from build123d import *

# Parameters (mm, degrees)
ESQUISSE1_W                               = 256
ESQUISSE1_H                               = 100
T_LE_DE_BASE_PLI_E1_DEPTH                 = 10
ESQUISSE15_W                              = 256
ESQUISSE15_H                              = 10
BOSS_EXTRU_3_DEPTH                        = 10
ENL_V_MAT_EXTRU_1_REACH                   = 277.02
ESQUISSE9_R                               = 39
SKETCH7_W                                 = 10
SKETCH7_H                                 = 55
EXTRUDE2_DEPTH                            = 10
SKETCH8_W                                 = 40
SKETCH8_H                                 = 200
EXTRUDE3_DEPTH                            = 10
ESQUISSE11_W                              = 15
ESQUISSE11_H                              = 10
BOSS_EXTRU_2_DEPTH                        = 10
TROU_POUR_TARAUDAGE_POUR_TROU_TARAUD_M1_D = 14
CHANFREIN1_SIZE                           = 2
TAB_START                                 = -10
TAB_AND_SLOT_TAB1_DEPTH                   = 10
DIAM_TRE_DU_PER_AGE_2_0_2_1_D             = 2
ENL_V_START                               = -10
ESQUISSE19_W                              = 78
ESQUISSE19_H                              = 10
ENL_V_MAT_EXTRU_2_DEPTH                   = 10


# Read off the part's stored shape, not the designer's step: Tab and Slot-Tab1
# Sheet-metal steps are written as plain solids
with BuildPart() as part:
    # Esquisse1 → Tôle de base pliée1 (new body)
    with BuildSketch(Plane.XY):
        with Locations((128, 50)):
            Rectangle(ESQUISSE1_W, ESQUISSE1_H)
    extrude(amount=-T_LE_DE_BASE_PLI_E1_DEPTH)

    # Esquisse15 → Boss.-Extru.3 (add)
    with BuildSketch(Plane.XY):
        with Locations((128, -5)):
            Rectangle(ESQUISSE15_W, ESQUISSE15_H)
    extrude(amount=-BOSS_EXTRU_3_DEPTH)

    # Esquisse9 → Enlèv. mat.-Extru.1 (cut, up to next)
    with BuildSketch(Plane.XY, mode=Mode.PRIVATE) as enl_v_mat_extru_1_sk1:
        with Locations((71, 0)):
            Circle(ESQUISSE9_R)
    enl_v_mat_extru_1_tool1 = extrude(enl_v_mat_extru_1_sk1.sketch, amount=-ENL_V_MAT_EXTRU_1_REACH, mode=Mode.PRIVATE) & part.part
    # Esquisse9 → Enlèv. mat.-Extru.1 (cut, up to next)
    with BuildSketch(Plane.XY, mode=Mode.PRIVATE) as enl_v_mat_extru_1_sk2:
        with Locations((185, 0)):
            Circle(ESQUISSE9_R)
    enl_v_mat_extru_1_tool2 = extrude(enl_v_mat_extru_1_sk2.sketch, amount=-ENL_V_MAT_EXTRU_1_REACH, mode=Mode.PRIVATE) & part.part
    add(enl_v_mat_extru_1_tool1.solids().sort_by_distance((71, 0, 0))[0], mode=Mode.SUBTRACT)
    add(enl_v_mat_extru_1_tool2.solids().sort_by_distance((185, 0, 0))[0], mode=Mode.SUBTRACT)

    # Sketch7 → Extrude2 (add)
    with BuildSketch(Plane.XY):
        with Locations((-5, 72.5)):
            Rectangle(SKETCH7_W, SKETCH7_H)
        with Locations((261, 72.5)):
            Rectangle(SKETCH7_W, SKETCH7_H)
    extrude(amount=-EXTRUDE2_DEPTH)

    # Sketch8 → Extrude3 (add)
    with BuildSketch(Plane.XY):
        with Locations((-30, 0)):
            Rectangle(SKETCH8_W, SKETCH8_H)
        with Locations((286, 0)):
            Rectangle(SKETCH8_W, SKETCH8_H)
    extrude(amount=-EXTRUDE3_DEPTH)

    # Esquisse11 → Boss.-Extru.2 (add)
    with BuildSketch(Plane.XZ.offset(100)):
        with Locations((-42.5, -5)):
            Rectangle(ESQUISSE11_W, ESQUISSE11_H)
        with Locations((298.5, -5)):
            Rectangle(ESQUISSE11_W, ESQUISSE11_H)
    extrude(amount=BOSS_EXTRU_2_DEPTH)

    # Trou pour taraudage pour trou taraudé M161 (through all)
    with Locations(Plane.XY):
        with Locations((71, 74), (185, 74)):
            Hole(TROU_POUR_TARAUDAGE_POUR_TROU_TARAUD_M1_D / 2)

    # Chanfrein1
    chanfrein1_edges = [part.edges().sort_by_distance(p)[0] for p in [
        (-35, -110, -5),
        (291, -110, -5),
        (0, -10, -5),
        (256, -10, -5),
    ]]
    chamfer(chanfrein1_edges, length=CHANFREIN1_SIZE)

    # Tab and Slot-Tab1 outline → Tab and Slot-Tab1 (add)
    with BuildSketch(Plane.XY.offset(TAB_START)):
        Polygon((50, 109), (49, 110), (21, 110), (20, 109), (20, 100), (50, 100), align=None)
        Polygon((206, 109), (206, 100), (236, 100), (236, 109), (235, 110), (207, 110), align=None)
        Polygon((113, 109), (113, 100), (143, 100), (143, 109), (142, 110), (114, 110), align=None)
    extrude(amount=TAB_AND_SLOT_TAB1_DEPTH)

    # Diamètre du perçage Ø2.0 (2)1 (through all)
    with Locations(Plane.XY):
        with Locations((-35, -100)):
            diam_tre_du_per_age_2_0_2_1 = Hole(DIAM_TRE_DU_PER_AGE_2_0_2_1_D / 2)

    # Répét. par esquisse1: Diamètre du perçage Ø2.0 (2)1 at 11 more places
    with Locations((54, 200, 0), (86, 200, 0), (147, 200, 0), (179, 200, 0), (240, 200, 0), (272, 200, 0), (301, 145, 0), (291, 145, 0), (326, 0, 0), (35, 145, 0), (25, 145, 0)):
        add(diam_tre_du_per_age_2_0_2_1, mode=Mode.SUBTRACT)

    # Esquisse19 → Enlèv. mat.-Extru.2 (cut)
    with BuildSketch(Plane.XY.offset(ENL_V_START)):
        with Locations((71, -5)):
            Rectangle(ESQUISSE19_W, ESQUISSE19_H)
        with Locations((185, -5)):
            Rectangle(ESQUISSE19_W, ESQUISSE19_H)
    extrude(amount=ENL_V_MAT_EXTRU_2_DEPTH, mode=Mode.SUBTRACT)


solid = part.part
Read the model definition and answer for the solid it produces. Units are mm, in the model's axes. A direction names the side the tool comes from. Give positions to 0.01 mm unless a question says otherwise; leave off trailing zeros. Write each loop counter-clockwise with the first axis right and the second up, starting at its lowest first coordinate (ties: lowest second). Pieces come first, ordered by that corner, then holes. Notation, with made-up numbers: (-1.75, 1) - (17.25, 1) arc R25 cw to (17.25, 17) - close; hole circle Ø9 at (-6, 48). An arc over 180 degrees is marked (long way). Use CSV: the item, a comma, the result in double quotes. Start each with the question number.
Item 1: The part is cut by section C-C, the plane z = -7.5. Count the separate pieces of the cut face and the enclosed holes in it, and give its area (3 significant figures).
Item 2: Flat-ended cylindrical pins translate along their axes: P1, Ø22.5, axis at x = 71, y = 74, coming from the -Z side; P2, Ø3, axis at x = 131.5, z = -4, coming from the -Y side; P3, Ø2.5, axis at y = 103, z = -3.5, coming from the -X side; P4, Ø4.5, axis at y = 104, z = -5, coming from the +X side. Find the tip coordinate at first contact, or state that the pin passes through.
Item 3: The part is cut by section A-A, the plane y = -45. Give the vertices of the cut face in (x, z).
Item 4: For faces 1 (the flat face through (128, 110, -5)), 2 (the flat face through (50, 104, -5)), 3 (the flat face through (-16, 100, -5)), 4 (the flat face through (32, -5, -5)), 5 (the flat face through (272, 100, -5)), determine the directions among +Z, -Z, +X, -X, +Y, -Y from which every point of the face is accessible in a straight line to the end or side of a thin tool.
Item 5: The part is cut by section D-D, the plane x = 162.5. Give the vertices of the cut face in (y, z).
Item 6: Consider line 1 (X direction, y = 75, z = -4); line 2 (X direction, y = 101, z = -7); line 3 (Y direction, x = 71, z = -4). Determine where each line is inside the solid, lowest interval first.
Item 7: The mould has two halves that part along Y. Classify faces 6 (the cylindrical face through (178.323, 76.103, -5.07)), 7 (the flat face through (239, -10, -5)), 8 (the flat face through (224, -5, -5)): pulls with the +Y half, pulls with the -Y half, needs draft (parallel to the pull), parting line crosses it, or undercut.
Item 8: The part is cut by section B-B, the plane x = 71. Give the vertices of the cut face in (y, z), and give its area (3 significant figures).
Taken from the geometry:
1,separate pieces,"1"
1,enclosed holes,"2"
1,area,"39,800 mm2"
2,P1,"z = -10"
2,P2,"y = -10"
2,P3,"x = 20"
2,P4,"x = 236"
3,outline,"(-50, -10) - (-10, -10) - (-10, 0) - (-50, 0) - close; (266, -10) - (306, -10) - (306, 0) - (266, 0) - close"
4,face 1,"+Z, -Z, +X, -X, +Y"
4,face 2,"+Z, -Z, +Y"
4,face 3,"+Z, -Z, -X, +Y"
4,face 4,"+Z, -Z, -Y"
4,face 5,"+Z, -Z, +X, +Y"
5,outline,"(31.86, -10) - (100, -10) - (100, 0) - (31.86, 0) - close"
6,line 1,"-50 to 64.07, 77.93 to 178.07, 191.93 to 306"
6,line 2,"20 to 50, 113 to 143, 206 to 236"
6,line 3,"39 to 67, 81 to 100"
7,face 6,"undercut"
7,face 7,"pulls with the -Y half"
7,face 8,"needs draft"
8,outline,"(39, -10) - (67, -10) - (67, 0) - (39, 0) - close; (81, -10) - (100, -10) - (100, 0) - (81, 0) - close"
8,area,"470 mm2"
